Can you work these out from the model? Positions are in its coordinate system, mm. A direction names the side the tool comes from. Round coordinates to 2 decimals unless told otherwise and drop trailing zeros. Order: outer loops, then holes, each group sorted by start corner. A loop starts at its lowest first (then second) coordinate and runs counter-clockwise, first axis right, second up. Notation, with made-up numbers: (89, 5.5) -> (125, 5.5) arc R22 ccw to (125, 41.5) -> close; hole circle Ø4 at (-30, 57.25). An arc over 180 degrees is marked (long way). Use a Markdown table: item, result. Add a question column.
Q1. If we section it at B-B on x = 57.5: List the corners of the cut face in (y, z) for me (3 decimals), plus the area to 3 significant figures.
Q2. If we section it at C-C on y = 20.5: Give the number of separate pieces and of enclosed holes in the cut face, plus the area to 3 significant figures.
Q3. I need wall thicknesses on line 1 along X through (y, z) = (3, 10.25); line 2 along X through (y, z) = (19.5, 3.5); line 3 along X through (y, z) = (21, 5.25). Which ranges of each line are inside material? Lowest first, please. Write a range as [from, to].
Q4. For faces 1 (the face through (-33.804, -11.305, 7.2)), 2 (the face through (-52.451, 22, 8)), which set-ups out of +Z, -Z, +X, -X, +Y, -Y let a thin tool reach every point of the face, with its end or its side?
Q5. I'm going to push flat-ended pins straight in: pin 1 Ø1 at (y, z) = (7, 9) entering from -X; pin 2 Ø2.5 at (y, z) = (20, 7.5) entering from +X; pin 3 Ø1.5 at (y, z) = (19, 8) entering from -X; pin 4 Ø4 at (x, y) = (57, -9) entering from -Z. Where does each tip first touch, or does it pass through?
Q6. If we section it at A-A on z = 8: List the corners of the cut face in (x, y) for me (3 decimals), plus the area to 3 significant figures.
Q7. We'd pull the mould along X, two halves only. Please class faces 3 (the face through (81.273, 10.03, 7.2)), 4 (the face through (42.799, 12, 8)), 5 (the face through (-0.02, -14.605, 7.2)), 6 (the face through (47.7, 11.7, 1.6)): +X half, -X half, draft (parallel to the pull), parting line (faces both ways), or undercut.
```python
from build123d import *

# Parameters (mm, degrees)
F0_R     = 9.525
F0_R_2   = 12.7
F1_DEPTH = 15.875
F3_DEPTH = 31.75
F4_SIZE  = 1.27


with BuildPart() as f1:
    # F0 (on Top) → F1 (new body)
    with BuildSketch(Plane.XY):
        with BuildLine():
            Line((63.5, 27.305), (-63.5, 27.305))
            ThreePointArc((-63.5, 27.305), (-81.258035, 10.408506), (-65.264829, -8.167195))
            Line((-65.264829, -8.167195), (-1.449681, -14.532875))
            ThreePointArc((-1.449681, -14.532875), (0, -14.605), (1.449681, -14.532875))
            Line((1.449681, -14.532875), (65.264829, -8.167195))
            ThreePointArc((65.264829, -8.167195), (81.258035, 10.408506), (63.5, 27.305))
        make_face()
        Circle(F0_R, mode=Mode.SUBTRACT)
        with Locations((-63.5, 9.525)):
            Circle(F0_R_2, mode=Mode.SUBTRACT)
        with Locations((63.5, 9.525)):
            Circle(F0_R_2, mode=Mode.SUBTRACT)
    extrude(amount=F1_DEPTH)

    # F2 (on face) → F3 (cut)
    with BuildSketch(Plane(origin=(0, 27.305, 0), x_dir=(-1, 0, 0), z_dir=(0, 1, 0))):
        with BuildLine():
            Line((52.451, 6.4262), (52.451, 9.4488))
            ThreePointArc((52.451, 9.4488), (47.625, 14.2748), (42.799, 9.4488))
            Line((42.799, 9.4488), (42.799, 6.4262))
            ThreePointArc((42.799, 6.4262), (47.625, 1.6002), (52.451, 6.4262))
        make_face()
        with BuildLine():
            ThreePointArc((-42.799, 9.4488), (-47.625, 14.2748), (-52.451, 9.4488))
            Line((-52.451, 9.4488), (-52.451, 6.4262))
            ThreePointArc((-52.451, 6.4262), (-47.625, 1.6002), (-42.799, 6.4262))
            Line((-42.799, 6.4262), (-42.799, 9.4488))
        make_face()
    extrude(amount=-F3_DEPTH, mode=Mode.SUBTRACT)

    # F4
    f4_edges = [f1.edges().sort_by_distance(p)[0] for p in [
        (-81.258035, 10.408506, 15.875),
    ]]
    chamfer(f4_edges, length=F4_SIZE)


solid = f1.part
```
Answer below:
| question | item | result |
|---|---|---|
| 1 | outline | (-8.942, 0) -> (-1.668, 0) -> (-1.668, 15.875) -> (-7.665, 15.875) -> (-8.942, 14.605) -> close; (20.718, 0) -> (27.305, 0) -> (27.305, 14.605) -> (26.035, 15.875) -> (20.718, 15.875) -> close |
| 1 | area | 218 mm² |
| 2 | separate pieces | 3 |
| 2 | enclosed holes | 2 |
| 2 | area | 1,850 mm² |
| 3 | line 1 | [-80.04, -74.4], [-52.6, -52.38], [-42.87, -9.04], [9.04, 42.87], [52.38, 52.6], [74.4, 80.04] |
| 3 | line 2 | [-78.22, -71.36], [-55.64, -51.46], [-43.79, 43.79], [51.46, 55.64], [71.36, 78.22] |
| 3 | line 3 | [-77.08, -68.94], [-58.06, -52.31], [-42.94, 42.94], [52.31, 58.06], [68.94, 77.08] |
| 4 | face 1 | +Z, -Z, -X, -Y |
| 4 | face 2 | +Y |
| 5 | pin 1 | x = -81.16 |
| 5 | pin 2 | x = 78.7 |
| 5 | pin 3 | x = -78.99 |
| 5 | pin 4 | z = 0 |
| 6 | outline | (-65.265, -8.167) -> (-1.45, -14.533) arc R14.605 ccw to (1.45, -14.533) -> (65.265, -8.167) arc R17.78 ccw to (63.5, 27.305) -> (52.451, 27.305) -> (52.451, 15.787) arc R12.7 cw (long way) to (52.451, 3.263) -> (52.451, -4.445) -> (42.799, -4.445) -> (42.799, 27.305) -> (-42.799, 27.305) -> (-42.799, -4.445) -> (-52.451, -4.445) -> (-52.451, 3.263) arc R12.7 cw (long way) to (-52.451, 15.787) -> (-52.451, 27.305) -> (-63.5, 27.305) arc R17.78 ccw to start; hole circle Ø19.05 at (0, 0) |
| 6 | area | 4,040 mm² |
| 7 | face 3 | +X half |
| 7 | face 4 | undercut |
| 7 | face 5 | parting line |
| 7 | face 6 | undercut |
